from build123d import *

# Parameters (mm, degrees)
EXTRUDE_1_DEPTH     = 18.35
CUT_EXTRUDE_1_DEPTH = 4
SHELL_START         = -16.36
SHELL_1_DEPTH       = 32.72
SKETCH_8_R          = 2.5
SKETCH_8_R_2        = 1.25
EXTRUDE_4_DEPTH     = 7.51
FILLET_1_R          = 0.7
SKETCH_10_W         = 8.837744534
SKETCH_10_H         = 38.466628308
SKETCH_10_W_2       = 9.721518987
SKETCH_10_H_2       = 38.024741082
CUT_EXTRUDE_2_DEPTH = 4
EXTRUDE_5_DEPTH     = 1.5
EXTRUDE_6_DEPTH     = 1.5


# Read off the part's stored shape, not the designer's step: the shell step
with BuildPart() as part:
    # Sketch 1 → Extrude 1 (new, symmetric)
    with BuildSketch(Plane(origin=(0, 0, 0), x_dir=(0, 0, -1), z_dir=(1, 0, 0))):
        Polygon((-13.5, 44), (0, 43.5), (0, -43.5), (-13.5, -44), align=None)
    extrude(amount=EXTRUDE_1_DEPTH, both=True)

    # Sketch 2 → Cut-Extrude 1 (cut)
    with BuildSketch(Plane(origin=(0, 0, 0), x_dir=(-1, 0, 0), z_dir=(0, 0, -1))):
        Polygon((-18.35, 17.65), (-9.3, 17.65), (-9.3, 20), (-16.35, 20), (-16.35, 42), (16.35, 42), (16.35, 20), (9.3, 20), (9.3, 17.65), (18.35, 17.65), (18.35, -17.65), (16.35, -17.65), (16.35, -42), (10, -42), (10, -19.65), (11.35, -19.65), (11.35, -17.65), (6, -17.65), (6, -39.65), (7.5, -39.65), (7.5, -44), (-7.5, -44), (-7.5, -39.65), (-6, -39.65), (-6, -17.65), (-11.35, -17.65), (-11.35, -19.65), (-10, -19.65), (-10, -42), (-16.35, -42), (-16.35, -17.65), (-18.35, -17.65), align=None)
    extrude(amount=-CUT_EXTRUDE_1_DEPTH, mode=Mode.SUBTRACT)

    # Shell 1 outline → Shell 1 (cut)
    with BuildSketch(Plane.YZ.offset(SHELL_START)):
        Polygon((-42.008635584, 13.5), (-41.730487436, 5.99), (41.730487436, 5.99), (42.008635584, 13.5), align=None)
    extrude(amount=SHELL_1_DEPTH, mode=Mode.SUBTRACT)

    # Sketch 8 → Extrude 4 (add)
    # profile 1 of 2: a face of its own
    with BuildSketch(Plane.XY.offset(5.99)):
        with Locations(Location((10.35, 25.5, 0), (0, 0, 180))):
            Circle(SKETCH_8_R)
        with Locations(Location((10.35, 25.5, 0), (0, 0, 180))):
            Circle(SKETCH_8_R_2, mode=Mode.SUBTRACT)
    # profile 2 of 2: a face of its own
    with BuildSketch(Plane.XY.offset(5.99)):
        with Locations(Location((-10.35, -25.5, 0), (0, 0, 180))):
            Circle(SKETCH_8_R)
        with Locations(Location((-10.35, -25.5, 0), (0, 0, 180))):
            Circle(SKETCH_8_R_2, mode=Mode.SUBTRACT)
    extrude(amount=EXTRUDE_4_DEPTH)

    # Fillet 1
    fillet_1_edges = [part.edges().sort_by_distance(p)[0] for p in [
        (17.35, -17.65, 0),
        (-18.35, -43.75, 6.75),
        (-18.35, -30.575, 0),
        (-18.35, 0, 4),
        (-18.35, 30.575, 0),
        (18.35, -43.75, 6.75),
        (18.35, -30.575, 0),
        (18.35, -17.65, 2),
        (18.35, 0, 4),
        (18.35, 17.65, 2),
        (18.35, 30.575, 0),
        (-18.35, 43.75, 6.75),
        (0, 43.5, 0),
        (18.35, 43.75, 6.75),
        (-12.925, -43.5, 0),
        (12.925, -43.5, 0),
        (-18.35, 17.65, 2),
    ]]
    fillet(fillet_1_edges, radius=FILLET_1_R)

    # Sketch 10 → Cut-Extrude 2 (cut, symmetric)
    with BuildSketch(Plane(origin=(0, 0, 0), x_dir=(1, 0, 0), z_dir=(0, 1, 0))):
        with Locations((-20.778872267, 0)):
            Rectangle(SKETCH_10_W, SKETCH_10_H)
        with Locations((21.220759494, 0)):
            Rectangle(SKETCH_10_W_2, SKETCH_10_H_2)
    extrude(amount=CUT_EXTRUDE_2_DEPTH, both=True, mode=Mode.SUBTRACT)


with BuildPart() as body_2:
    # Sketch 11 → Extrude 5 (new body)
    with BuildSketch(Plane(origin=(-16.36, 0, 0), x_dir=(0, 0, -1), z_dir=(1, 0, 0))):
        Polygon((-5.99, 5.5), (-10.99, 5.5), (-10.99, 3), (-18.99, 3), (-18.99, -3), (-10.99, -3), (-10.99, -5.5), (-5.99, -5.5), align=None)
    extrude_5 = extrude(amount=EXTRUDE_5_DEPTH)



with BuildPart() as part_1:
    add(part.part)

    # Mirror 2: Extrude 5 across plane
    add(extrude_5.mirror(Plane(origin=(0, 0, 0), x_dir=(0, 0, 1), z_dir=(1, 0, 0))))


with BuildPart() as body_2_1:
    add(body_2.part)

    add(part_1.part)  # Extrude 6 merges part
    # Sketch 12 → Extrude 6 (add)
    with BuildSketch(Plane.XY.offset(13.5)):
        Polygon((-16.36, 4), (-16.36, 42.008635584), (16.36, 42.008635584), (16.36, 4), (17.36, 4), (17.36, 43.008635584), (-17.36, 43.008635584), (-17.36, 4), align=None)
    extrude_6 = extrude(amount=EXTRUDE_6_DEPTH)

    # Mirror 3: Extrude 6 across plane
    add(extrude_6.mirror(Plane.ZX))


solid = body_2_1.part
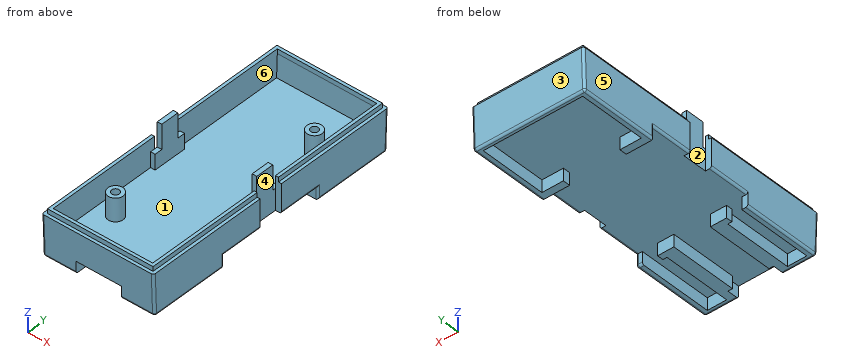
Geometry check sheet. Reference: the model listing, model coordinates, mm. Face numbers are marked on the shaded views. A direction names the side the tool comes from. Round coordinates to 2 decimals unless told otherwise and drop trailing zeros. Loops run counter-clockwise (first coordinate to the right, second up) from the corner with the lowest first, then second, coordinate; pieces in that order, holes last. Notation, with made-up numbers: (40, -5.5) - (45, -5.5) arc R35 cw to (45, 30.5) - close; hole circle Ø11 at (8.5, 67). An arc over 180 degrees is marked (long way). One line per question, with ' | ' between items. Start each with the question number.
1. Cross-section at A-A on z = 17. Record the cut outline in (x, y), then the cut area to 3 significant figures.
2. Cross-section at B-B on y = -8. Record the cut outline in (x, z), then the cut area to 3 significant figures.
3. Scan lines: line 1 (X direction, y = -25.5, z = 8); line 2 (X direction, y = 25.5, z = 12); line 3 (Y direction, x = 6.5, z = 14.5). Record each from-to range of solid material in increasing order. Write a range as [from, to].
4. Depth check by flat-ended pin: pin 1 (3 mm diameter, centred on x = -10.35, y = -25.5, fed in from +Z); pin 2 (1.5 mm diameter, centred on x = 6.5, z = 9, fed in from +Y); pin 3 (2 mm diameter, centred on x = -14, z = 1, fed in from +Y); pin 4 (2 mm diameter, centred on x = 9, z = 16.5, fed in from +Y). Enter the tip coordinate at first touch or a pass-through.
5. Cross-section at D-D on z = 8.25. State how many separate pieces and enclosed holes the cut face has, then the cut area to 3 significant figures.
6. Tool access check on the marked faces 4, 5 and 6. Record the directions out of +Z, -Z, +X, -X, +Y, -Y that give a thin tool (end or side, any length) a straight path to the whole face; none if there is none.
7. Draft check along X on the marked faces 1, 2 and 3. Enter one of: released by +X, released by -X, zero draft, split by the parting line, or undercut.
Taken from the geometry:
1) outline: (-16.36, -3) - (-14.86, -3) - (-14.86, 3) - (-16.36, 3) - close; (14.86, -3) - (16.36, -3) - (16.36, 3) - (14.86, 3) - close | area: 18.0 mm²
2) outline: (-18.35, 4.7) arc R0.7 ccw to (-17.65, 4) - (17.65, 4) arc R0.7 ccw to (18.35, 4.7) - (18.35, 13.5) - (17.36, 13.5) - (17.36, 15) - (16.36, 15) - (16.36, 5.99) - (-16.36, 5.99) - (-16.36, 15) - (-17.36, 15) - (-17.36, 13.5) - (-18.35, 13.5) - close | area: 106 mm²
3) line 1: [-18.35, -16.36], [-12.85, -11.6], [-9.1, -7.85], [16.36, 18.35] | line 2: [-18.35, -16.36], [7.85, 9.1], [11.6, 12.85], [16.36, 18.35] | line 3: [-43.01, -42.01], [42.01, 43.01]
4) pin 1: z = 13.5 | pin 2: y = 43.86 | pin 3: y = 43.57 | pin 4: through
5) separate pieces: 3 | enclosed holes: 3 | area: 509 mm²
6) face 4: +Z, -Z, +X | face 5: +Z, -Z, -X, +Y, -Y | face 6: +Z
7) face 1: undercut | face 2: released by -X | face 3: zero draft
